Drawing for the job (mm, zero at the part's lowest x, y, z). Give positions to 0.01 mm unless a question says otherwise; leave off trailing zeros. Order: outer loops, then holes, each group sorted by start corner. A loop starts at its lowest first (then second) coordinate and runs counter-clockwise, first axis right, second up. Notation, with made-up numbers: (-31.75, -2.75) - (-13.75, -2.75) arc R18 ccw to (-13.75, 23.25) - close; hole circle Ø3 at (88, -2). An arc over 180 degrees is marked (long way). Use a Markdown table: item, result. Add a question column.
(1) Wall check: line 1 (Z direction, x = 57.15, y = 1.1); line 2 (X direction, y = 1.5, z = 19.05); line 3 (X direction, y = 0.8, z = 6.35). Give the ranges that are in metal, low to high.
(2) Slice it at D-D (z = 6.35). Write the cut outline in (x, y) (1 decimal).
(3) Slice it at C-C (y = 1.85). Count the separate pieces of the cut face and the enclosed holes in it, then the cut area to 3 significant figures.
(4) Flat gauge pin, fed straight in: pin 1 (1.6 mm diameter, centred on y = 1.5, z = 5, fed in from +X). Where does the tip first touch, or does it go through?
(5) Slice it at A-A (x = 44.45). Write the cut outline in (y, z) (1 decimal), then the cut area to 3 significant figures.
(6) Slice it at B-B (z = 19.05). Write the cut outline in (x, y) (1 decimal), then the cut area to 3 significant figures.
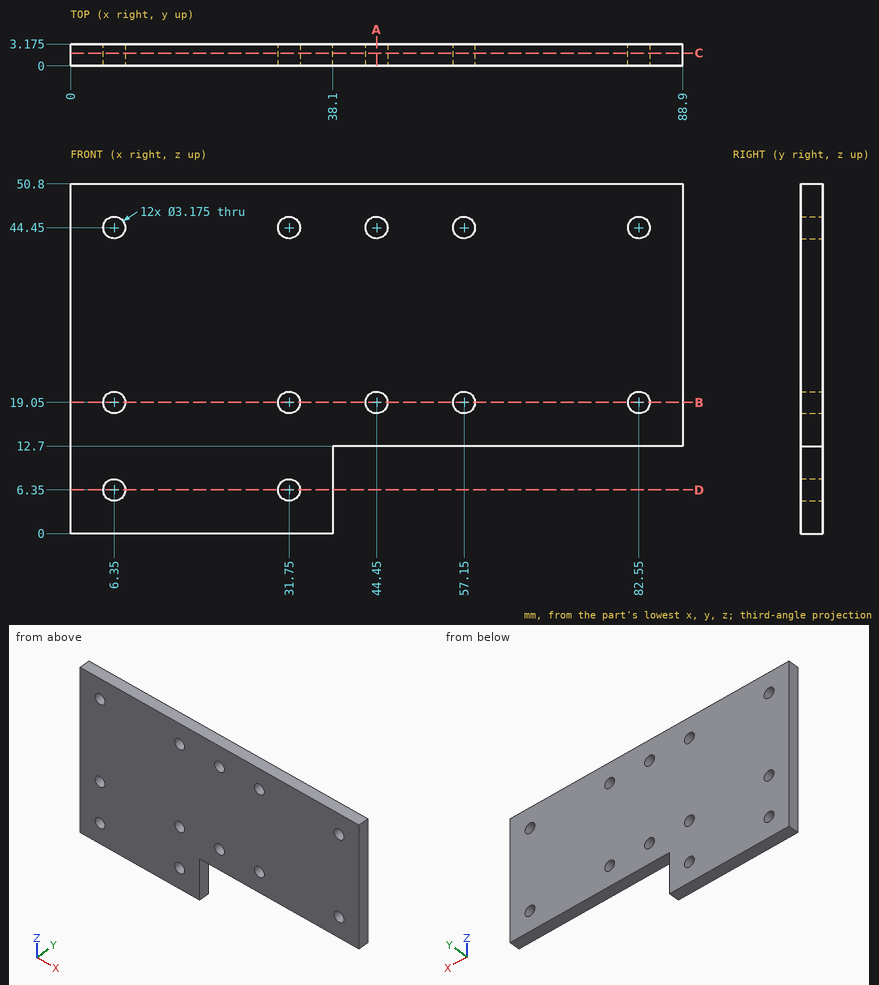
Solution:
| question | item | result |
|---|---|---|
| 1 | line 1 | 12.7 to 17.46, 20.64 to 42.86, 46.04 to 50.8 |
| 1 | line 2 | 0 to 4.76, 7.94 to 30.16, 33.34 to 42.86, 46.04 to 55.56, 58.74 to 80.96, 84.14 to 88.9 |
| 1 | line 3 | 0 to 4.76, 7.94 to 30.16, 33.34 to 38.1 |
| 2 | outline | (0, 0) - (4.8, 0) - (4.8, 3.2) - (0, 3.2) - close; (7.9, 0) - (30.2, 0) - (30.2, 3.2) - (7.9, 3.2) - close; (33.3, 0) - (38.1, 0) - (38.1, 3.2) - (33.3, 3.2) - close |
| 3 | separate pieces | 1 |
| 3 | enclosed holes | 12 |
| 3 | area | 3,780 mm2 |
| 4 | pin 1 | x = 38.1 |
| 5 | outline | (0, 12.7) - (3.2, 12.7) - (3.2, 17.5) - (0, 17.5) - close; (0, 20.6) - (3.2, 20.6) - (3.2, 42.9) - (0, 42.9) - close; (0, 46) - (3.2, 46) - (3.2, 50.8) - (0, 50.8) - close |
| 5 | area | 101 mm2 |
| 6 | outline | (0, 0) - (4.8, 0) - (4.8, 3.2) - (0, 3.2) - close; (7.9, 0) - (30.2, 0) - (30.2, 3.2) - (7.9, 3.2) - close; (33.3, 0) - (42.9, 0) - (42.9, 3.2) - (33.3, 3.2) - close; (46, 0) - (55.6, 0) - (55.6, 3.2) - (46, 3.2) - close; (58.7, 0) - (81, 0) - (81, 3.2) - (58.7, 3.2) - close; (84.1, 0) - (88.9, 0) - (88.9, 3.2) - (84.1, 3.2) - close |
| 6 | area | 232 mm2 |
